Input: part model. Units: mm. Frame: model coordinates. A direction names the side the tool comes from. Coordinates: 2 decimals unless noted, no trailing zeros. Write each loop counter-clockwise with the first axis right and the second up, starting at its lowest first coordinate (ties: lowest second). Pieces come first, ordered by that corner, then holes. Notation, with made-up numbers: M 88.5,8.25 L 94.5,8.25 A11 cw 94.5,19.25 Z; hole C 32,30 d7. An arc over 180 degrees is marked long. Use one line per item in the form item = value.
from build123d import *

# Parameters (mm, degrees)
F0_R     = 5.1
F1_DEPTH = 30
F2_DEPTH = 22.5
F3_R     = 5


with BuildPart() as f1:
    # F0 (on Right) → F1 (new body, symmetric)
    with BuildSketch(Plane.YZ):
        with BuildLine():
            ThreePointArc((24.8170878902, -397.7473182194), (23.8345837656, -395.9821311786), (22.4412201864, -394.5193469909))
            ThreePointArc((22.4412201864, -394.5193469909), (10.1667790366, -404.1596589088), (25.391624, -400.724311))
            ThreePointArc((25.391624, -400.724311), (25.2466768681, -399.2083477949), (24.8170878902, -397.7473182194))
        make_face()
        with Locations((17.391624, -400.724311)):
            Circle(F0_R, mode=Mode.SUBTRACT)
    extrude(amount=F1_DEPTH, both=True)

    # F0 (on Right) → F2 (join, symmetric)
    with BuildSketch(Plane.YZ):
        with BuildLine():
            Line((41.6709488454, -385.2116712139), (30.7416916961, -388.3455854761))
            Line((30.7416916961, -388.3455854761), (22.637896, -394.373063))
            Line((22.637896, -394.373063), (22.936297, -394.774257))
            ThreePointArc((22.936297, -394.774257), (25.2411173155, -396.1514104487), (27.8446650687, -395.4954474882))
            Line((27.8446650687, -395.4954474882), (41.6709488454, -385.2116712139))
        make_face()
        with BuildLine():
            Line((57.3466358684, -380.7167399976), (61.4554451408, -379.5385578207))
            Line((61.4554451408, -379.5385578207), (54.733396, -370.500928))
            Line((54.733396, -370.500928), (30.7416916961, -388.3455854761))
            Line((30.7416916961, -388.3455854761), (41.6709488454, -385.2116712139))
            Line((41.6709488454, -385.2116712139), (51.1139020687, -378.1881484882))
            ThreePointArc((51.1139020687, -378.1881484882), (53.7055684242, -377.5351807229), (55.999871, -378.906048))
            Line((55.999871, -378.906048), (57.3466358684, -380.7167399976))
        make_face()
        with BuildLine():
            Line((65.1262132866, -384.4738153538), (61.4554451408, -379.5385578207))
            Line((61.4554451408, -379.5385578207), (57.3466358684, -380.7167399976))
            Line((57.3466358684, -380.7167399976), (61.371102, -386.127535))
            ThreePointArc((61.371102, -386.127535), (62.3300853011, -387.0102243008), (63.5455334662, -387.4808357451))
            ThreePointArc((63.5455334662, -387.4808357451), (64.9729225904, -387.4475961696), (66.26827, -386.84708))
            Line((66.26827, -386.84708), (66.669464, -386.548678))
            Line((66.669464, -386.548678), (65.1262132866, -384.4738153538))
        make_face()
        Polygon((66.132787, -384.235166), (66.6175101107, -386.2796280266), (67.1738194665, -388.0992339037), (91.437887, -382.346447), (90.515105, -378.454343), align=None)
        with BuildLine():
            Line((66.001939903, -384.2661886412), (65.1262132866, -384.4738153538))
            Line((65.1262132866, -384.4738153538), (66.669464, -386.548678))
            Line((66.669464, -386.548678), (66.26827, -386.84708))
            ThreePointArc((66.26827, -386.84708), (64.9729225904, -387.4475961696), (63.5455334662, -387.4808357451))
            Line((63.5455334662, -387.4808357451), (67.055569, -388.12727))
            Line((67.055569, -388.12727), (66.6175101107, -386.2796280266))
            Line((66.6175101107, -386.2796280266), (66.001939903, -384.2661886412))
        make_face()
        Polygon((66.132787, -384.235166), (66.001939903, -384.2661886412), (66.6175101107, -386.2796280266), align=None)
        Polygon((67.1738194665, -388.0992339037), (66.6175101107, -386.2796280266), (67.055569, -388.12727), align=None)
        with BuildLine():
            Line((22.936297, -394.774257), (22.637896, -394.373063))
            Line((22.637896, -394.373063), (22.4412201864, -394.5193469909))
            ThreePointArc((22.4412201864, -394.5193469909), (23.8345837656, -395.9821311786), (24.8170878902, -397.7473182194))
            Line((24.8170878902, -397.7473182194), (27.8446650687, -395.4954474882))
            ThreePointArc((27.8446650687, -395.4954474882), (25.2411173155, -396.1514104487), (22.936297, -394.774257))
        make_face()
    extrude(amount=F2_DEPTH, both=True)

    # F3
    f3_edges = [f1.edges().sort_by_distance(p)[0] for p in [
        (22.5, 90.976496, -380.400395),
        (-22.5, 90.976496, -380.400395),
    ]]
    fillet(f3_edges, radius=F3_R)


solid = f1.part
(1) Section query B-B on x = -20.5. Return the cut outline in (y, z).
Computed:
outline = M 22.44,-394.52 A8 ccw long 24.82,-397.75 L 27.84,-395.5 L 51.11,-378.19 A3.49 cw 56,-378.91 L 61.37,-386.13 A3.5 ccw 63.55,-387.48 L 67.06,-388.13 L 90.46,-382.58 L 89.54,-378.69 L 65.13,-384.47 L 54.73,-370.5 L 22.64,-394.37 Z; hole C 17.39,-400.72 d10.2
(2) Pull-direction query (Y, two-part tool) for faces 3 (the cylindrical face through (-21.07, 89.51, -380.72)), 4 (the flat face through (0.32, 65.28, -387.8)), 5 (the flat face through (-30, 23, -401)); classes: pulls with the +Y half, pulls with the -Y half, needs draft (parallel to the pull), parting line crosses it, or undercut.
Computed:
face_3 = pulls with the +Y half
face_4 = undercut
face_5 = needs draft
(3) Section query D-D on x = 11. Return the cut outline in (y, z).
Computed:
outline = M 22.44,-394.52 A8 ccw long 24.82,-397.75 L 27.84,-395.5 L 51.11,-378.19 A3.49 cw 56,-378.91 L 61.37,-386.13 A3.5 ccw 63.55,-387.48 L 67.06,-388.13 L 91.44,-382.35 L 90.52,-378.45 L 65.13,-384.47 L 54.73,-370.5 L 22.64,-394.37 Z; hole C 17.39,-400.72 d10.2
(4) Set-up query: faces 1 (the cylindrical face through (0.315, 62.315, -387)), 2 (the cylindrical face through (21, 89.58, -380.7)). Return all of +Z, -Z, +X, -X, +Y, -Y with unobstructed straight access to the full face (end or side cutting, diameter ignored); none if empty.
Computed:
face_1 = -Z, +X, -X
face_2 = +Z, +X, +Y
(5) Line query: probe 1 along Y at (x, z) = (26, -400.5); probe 2 along Y at (x, z) = (2, -405); probe 3 along X at (y, z) = (47.5, -379). Output: solid intervals per line, ascending.
Computed:
probe_1 = 9.39 to 12.3, 22.49 to 25.39
probe_2 = 10.63 to 14.61, 20.17 to 24.15
probe_3 = -22.5 to 22.5
(6) Section query A-A on z = -403. Return the cut outline in (x, y), plus the area to 3 significant figures.
Computed:
outline = M -30,9.72 L 30,9.72 L 30,12.83 L -30,12.83 Z; M -30,21.96 L 30,21.96 L 30,25.06 L -30,25.06 Z
area = 373 mm^2
(7) Section query C-C on y = 15. Return the cut outline in (x, z), plus the area to 3 significant figures.
Computed:
outline = M -30,-408.36 L 30,-408.36 L 30,-405.23 L -30,-405.23 Z; M -30,-396.22 L 30,-396.22 L 30,-393.09 L -30,-393.09 Z
area = 376 mm^2
(8) First-contact query: pin 1 Ø8 at (x, y) = (6, 24) entering from +Z; pin 2 Ø8 at (x, z) = (24, -400.5) entering from +Y; pin 3 Ø6 at (x, y) = (-15, 56) entering from -Z. Flat tips, straight axial feed; report the tip coordinate or a pass-through.
Computed:
pin_1 = -390.38
pin_2 = 26.1
pin_3 = -382.94
